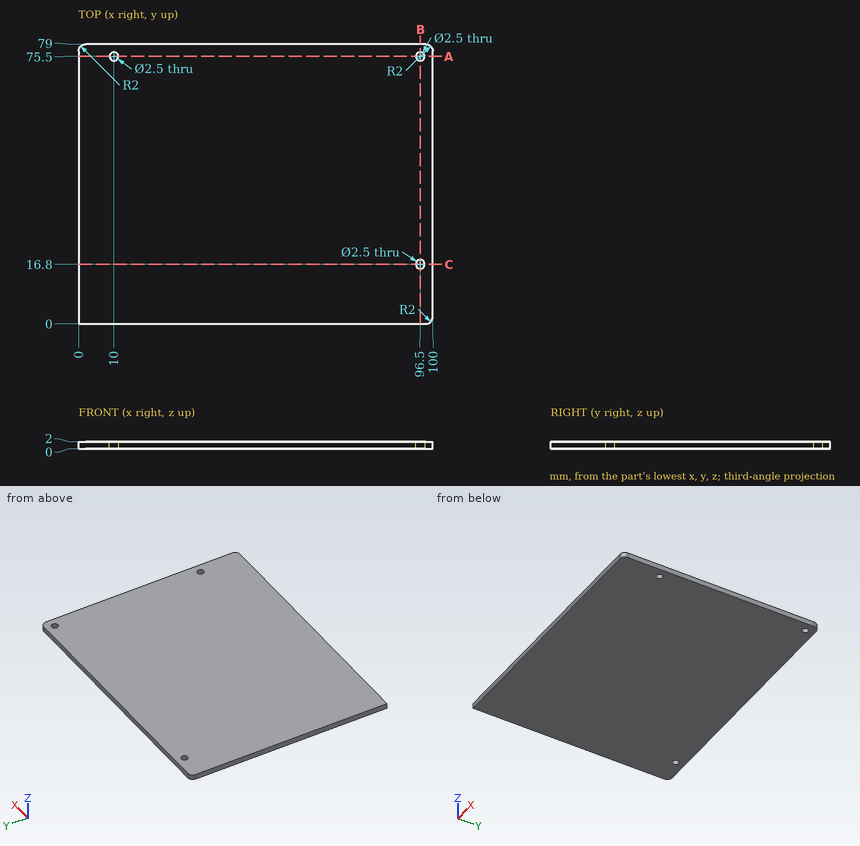
Could you check a few things on this drawing? It's one solid part, dimensions in mm from its lowest x, y, z. Round coordinates to 2 decimals unless told otherwise and drop trailing zeros. Write each loop counter-clockwise with the first axis right and the second up, starting at its lowest first coordinate (ties: lowest second). Pieces come first, ordered by that corner, then holes. Notation, with made-up numbers: (50, 87) -> (85, 87) arc R26 cw to (85, 103) -> close; hole circle Ø6 at (64, 41.25). An arc over 180 degrees is marked (long way). Use one line per item in the form item = value. Start each with the question number.
Q1. Imagine slicing it at C-C (y = 16.8). Please give me the cut outline in (x, z).
Q2. Imagine slicing it at B-B (x = 96.5). Please give me the cut outline in (y, z), then the cut area to 3 significant figures.
Q3. I'm going to push flat-ended pins straight in: P1, Ø3, axis at x = 10, y = 75.5, coming from the +Z side; P2, Ø2, axis at x = 96.5, y = 16.8, coming from the -Z side. Where does each tip first touch, or does it pass through?
Q4. Imagine slicing it at A-A (y = 75.5). Please give me the cut outline in (x, z).
Q5. If I drill on probe 1 along Y at (x, z) = (96.5, 1.4); probe 2 along X at (y, z) = (75.5, 0.8); probe 3 along Y at (x, z) = (10, 1.55), over which ranges is the centre line in solid material (lowest first)? Write a range as [from, to].
Worked out:
q1.outline = (0, 0) -> (95.25, 0) -> (95.25, 2) -> (0, 2) -> close; (97.75, 0) -> (100, 0) -> (100, 2) -> (97.75, 2) -> close
q2.outline = (0, 0) -> (15.55, 0) -> (15.55, 2) -> (0, 2) -> close; (18.05, 0) -> (74.25, 0) -> (74.25, 2) -> (18.05, 2) -> close; (76.75, 0) -> (79, 0) -> (79, 2) -> (76.75, 2) -> close
q2.area = 148 mm^2
q3.P1 = 2
q3.P2 = through
q4.outline = (0, 0) -> (8.75, 0) -> (8.75, 2) -> (0, 2) -> close; (11.25, 0) -> (95.25, 0) -> (95.25, 2) -> (11.25, 2) -> close; (97.75, 0) -> (100, 0) -> (100, 2) -> (97.75, 2) -> close
q5.probe_1 = [0, 15.55], [18.05, 74.25], [76.75, 79]
q5.probe_2 = [0, 8.75], [11.25, 95.25], [97.75, 100]
q5.probe_3 = [0, 74.25], [76.75, 79]
